from build123d import *

# Parameters (mm, degrees)
F1_DEPTH = 63.5
F2_DEPTH = 10.4775
F0_W     = 25.4
F0_H     = 19.05
F3_DEPTH = 25.4
F5_R     = 7.62


with BuildPart() as f1:
    # F0 (on Front) → F1 (new body, symmetric)
    with BuildSketch(Plane.XZ):
        Polygon((-41.275, -9.525), (41.275, -9.525), (41.275, 9.525), (22.225, 9.525), (-41.275, 9.525), align=None)
    extrude(amount=F1_DEPTH, both=True)

    # F0 (on Front) → F2 (join, symmetric)
    with BuildSketch(Plane.XZ):
        with BuildLine():
            add(Edge.make_bspline(
                [(-41.275, 9.525), (-24.2267409632, 30.0944438393), (5.5825358431, 60.821203998), (55.971666309, 61.9053164547)],
                knots=[0, 0, 0, 0, 110.6448027751, 110.6448027751, 110.6448027751, 110.6448027751], degree=3))
            Line((-41.275, 9.525), (22.225, 9.525))
            Line((22.225, 9.525), (22.225, 27.0002))
            ThreePointArc((22.225, 27.0002), (32.041147685, 51.2757259556), (55.971666309, 61.9053164547))
        make_face()
    extrude(amount=F2_DEPTH, both=True)

    # F0 (on Front) → F3 (join, symmetric)
    with BuildSketch(Plane.XZ):
        with BuildLine():
            Line((22.225, 9.525), (41.275, 9.525))
            Line((41.275, 9.525), (41.275, 27.0002))
            ThreePointArc((41.275, 27.0002), (45.9246798487, 38.2255201513), (57.15, 42.8752))
            Line((57.15, 42.8752), (60.325, 42.8752))
            Line((60.325, 42.8752), (60.325, 61.9252))
            Line((60.325, 61.9252), (57.15, 61.9252))
            add(Edge.make_bspline(
                [(55.971666309, 61.9053164547), (56.3632004506, 61.9137402364), (56.7559771249, 61.9203743088), (57.15, 61.9252)],
                knots=[110.6448027751, 110.6448027751, 110.6448027751, 110.6448027751, 111.5045361635, 111.5045361635, 111.5045361635, 111.5045361635], degree=3))
            ThreePointArc((55.971666309, 61.9053164547), (32.041147685, 51.2757259556), (22.225, 27.0002))
            Line((22.225, 27.0002), (22.225, 9.525))
        make_face()
        with Locations((73.025, 52.4002)):
            Rectangle(F0_W, F0_H)
    extrude(amount=F3_DEPTH, both=True)

    # F0 (on Front) → F4 (revolve)
    with BuildSketch(Plane.XZ):
        Polygon((85.725, 61.9252), (85.725, 42.8752), (85.725, 38.1), (111.125, 38.1), (111.125, 66.675), (85.725, 66.675), align=None)
    revolve(axis=Axis((85.725, 0, 52.3875), (0, 0, 1)))

    # F5
    f5_edges = [f1.edges().sort_by_distance(p)[0] for p in [
        (41.275, -63.5, 0),
        (-41.275, -63.5, 0),
        (41.275, 63.5, 0),
        (-41.275, 63.5, 0),
    ]]
    fillet(f5_edges, radius=F5_R)


solid = f1.part
CAD build for the part. Positions are in the model's coordinates, mm. A direction names the side the tool comes from. Round coordinates to 2 decimals unless told otherwise and drop trailing zeros. Write each loop counter-clockwise with the first axis right and the second up, starting at its lowest first coordinate (ties: lowest second). Pieces come first, ordered by that corner, then holes. Notation, with made-up numbers: M -30,73.5 L -15,73.5 A27 ccw -15,100.5 Z; hole C -11.5,64.25 d11. An arc over 180 degrees is marked long. Use a Markdown table: item, result. Add a question column.
1. Drill centre lines: probe 1 along Z at (x, y) = (41, -26.5) (3 decimals); probe 2 along Y at (x, z) = (30, 12); probe 3 along X at (y, z) = (-3, 38.5). Where is each one in solid material? Low to high.
2. 3-axis set-ups, long thin cutter, end or side, ignore diameter. For faces 1 (the face through (46, 25.4, 42)), 2 (the face through (8, 10.478, 30)), 3 (the face through (8, -10.478, 30)): which of +Z, -Z, +X, -X, +Y, -Y reach the whole face in a straight line?
3. Slice it at A-A on x = 74. Give the cut face in (y, z) (3 decimals).
4. Slice it at B-B on y = 27.5. Give the cut face in (x, z) (3 decimals).
5. Flat gauge pins, fed straight in: P1, Ø15.5, axis at x = 51, z = 46, coming from the +Y side; P2, Ø6, axis at x = 38.5, z = 58, coming from the -Y side; P3, Ø8, axis at y = 20, z = 17, coming from the -X side (3 decimals); P4, Ø16.5, axis at y = 20.5, z = 15.5, coming from the -X side (3 decimals). Where does each tip first touch, or does it go through?
6. Slice it at C-C on x = 93. Give the cut face in (y, z) (3 decimals), then the cut area to 3 significant figures.
7. Pull direction X, two halves, no side cores. Call faces 4 (the face through (85, 0, 66.675)), 5 (the face through (32.3, 17.83, 51.54)), 6 (the face through (60, 2, 42.875)): released by +X, released by -X, zero draft, split by the parting line, or undercut.
Reply:
| question | item | result |
|---|---|---|
| 1 | probe 1 | z = -9.525 to 9.525 |
| 1 | probe 2 | y = -25.4 to 25.4 |
| 1 | probe 3 | x = -11.62 to 46.21, 60.5 to 110.95 |
| 2 | face 1 | +Z, +X, -X, +Y |
| 2 | face 2 | +Z, -X, +Y |
| 2 | face 3 | +Z, -X, -Y |
| 3 | outline | M -25.4,42.875 L -22.532,42.875 L -22.532,38.1 L 22.532,38.1 L 22.532,42.875 L 25.4,42.875 L 25.4,61.925 L 22.532,61.925 L 22.532,66.675 L -22.532,66.675 L -22.532,61.925 L -25.4,61.925 Z |
| 4 | outline | M -41.275,-9.525 L 41.275,-9.525 L 41.275,9.525 L -41.275,9.525 Z |
| 5 | P1 | stops at y = 25.4 |
| 5 | P2 | stops at y = -25.4 |
| 5 | P3 | stops at x = 22.225 |
| 5 | P4 | stops at x = -41.275 |
| 6 | outline | M -24.336,38.1 L 24.336,38.1 L 24.336,66.675 L -24.336,66.675 Z |
| 6 | area | 1,390 mm^2 |
| 7 | face 4 | zero draft |
| 7 | face 5 | released by -X |
| 7 | face 6 | undercut |
